Design review of the part built by this model. Coordinates are the model's own, in mm. A direction names the side the tool comes from. Give positions to 0.01 mm unless a question says otherwise; leave off trailing zeros. Loops run counter-clockwise (first coordinate to the right, second up) from the corner with the lowest first, then second, coordinate; pieces in that order, holes last. Notation, with made-up numbers: (50, -17) - (108, -17) arc R23 ccw to (108, 5) - close; hole circle Ø6 at (4.25, 31.25). An arc over 180 degrees is marked (long way). Write each question's results on one line, items separated by ' | '.
Autodesk Inventor part; units mm, degrees
ref_plane "Work Plane1" through (-19.05, 0, 0) normal (1, 0, 0) x (0, 0, -1)
ref_plane "YZ Plane" through (0, 0, 0) normal (1, 0, 0) x (0, 1, 0)
ref_plane "XZ Plane" through (0, 0, 0) normal (0, 1, 0) x (-1, 0, 0)
sketch "Sketch2" plane through (0, 0, 0) normal (1, 0, 0) x (0, 1, 0)
  circle A0 centre (0, 0) radius 3.175
  dimension "d0" = 6.35
extrude "Extrusion1" add sketch "Sketch2" along normal mid plane 127
sketch "Sketch3" plane through (-63.5, 0, 0) normal (-1, 0, 0) x (0, 0, 1)
  circle A0 centre (0, 0) radius 12.7
  dimension "d3" = 25.4
extrude "Extrusion2" add sketch "Sketch3" against normal blind 6.35
sketch "Sketch4" plane through (-57.15, 0, 0) normal (1, 0, 0) x (0, 0, -1)
  line L0 (0, 4.572) -> (1.27, 4.572)
  line L1 (1.27, 4.572) -> (1.27, 2.9099)
  circle A0 centre (0, 0) radius 3.175
  line L2 (0, -17.78) -> (0, 17.78)
  line L3 (0, 4.572) -> (-1.27, 4.572)
  line L4 (-1.27, 4.572) -> (-1.27, 2.9099)
  line L5 (-4.572, 0) -> (-4.572, -1.27)
  line L6 (-4.572, 0) -> (-4.572, 1.27)
  line L7 (-4.572, 1.27) -> (-2.9099, 1.27)
  line L8 (-4.572, -1.27) -> (-2.9099, -1.27)
  line L9 (0, -4.572) -> (1.27, -4.572)
  line L10 (0, -4.572) -> (-1.27, -4.572)
  line L11 (-1.27, -4.572) -> (-1.27, -2.9099)
  line L12 (1.27, -4.572) -> (1.27, -2.9099)
  line L13 (4.572, 0) -> (4.572, 1.27)
  line L14 (4.572, 0) -> (4.572, -1.27)
  line L15 (4.572, -1.27) -> (2.9099, -1.27)
  line L16 (4.572, 1.27) -> (2.9099, 1.27)
  arc A1 (1.27, 2.9099) -> (-1.27, 2.9099) centre (0, 0) ccw
  arc A2 (2.9099, -1.27) -> (2.9099, 1.27) centre (0, 0) ccw
  arc A3 (-2.9099, 1.27) -> (-2.9099, -1.27) centre (0, 0) ccw
  arc A4 (-1.27, -2.9099) -> (1.27, -2.9099) centre (0, 0) ccw
  dimension "d7" = 1.27
  dimension "d10" = 360
  dimension "d15" = 1.397
extrude "Extrusion3" add sketch "Sketch4" along normal blind 76.2 contours L0 L1 A0 L2 | L2 A0 L4 L3 | L2 L10 L11 A0 | A0 L12 L9 L2 | L16 L13 L14 L15 A0 | A0 L8 L5 L6 L7
ref_plane "Work Plane1" through (-19.05, 0, 0) normal (1, 0, 0) x (0, 0, -1)
sketch "Sketch5" plane through (-19.05, 0, 0) normal (1, 0, 0) x (0, 0, -1)
  circle A0 centre (0, 0) radius 3.175
  circle A1 centre (0, 0) radius 5.4209
extrude "Extrusion4" cut sketch "Sketch5" against normal blind 38.1
properties part number "ShaftForWormGear" material "PBT Plastic"
Item 1: We need section B-B on x = -26. Give the boundary of the cut face in (y, z) (3 decimals).
Output values:
outline: circle Ø6.35 at (0, 0)
Item 2: We need section C-C on z = 6.25. Give the boundary of the cut face in (x, y), then the cut area to 3 significant figures.
Output values:
outline: (-63.5, -11.06) - (-57.15, -11.06) - (-57.15, 11.06) - (-63.5, 11.06) - close | area: 140 mm²
Item 3: Tool access review of faces 1 (the face through (0, 0, -4.572)), 2 (the face through (0, 4.572, 0)), 3 (the face through (0, 0, 4.572)), 4 (the face through (4.02, 2.513, 1.94)): name each direction out of +Z, -Z, +X, -X, +Y, -Y from which nothing blocks a thin tool from reaching the whole face with its end or side.
Output values:
face 1: -Z, +X, +Y, -Y | face 2: +Z, -Z, +X, +Y | face 3: +Z, +X, +Y, -Y | face 4: none
Item 4: Wall thickness on probe 1 along X at (y, z) = (0.75, -5.5); probe 2 along X at (y, z) = (-1, 3.25); probe 3 along Z at (x, y) = (4.5, -0.75): over which ranges is each line inside the solid? List them lowest first.
Output values:
probe 1: x = -63.5 to -57.15 | probe 2: x = -63.5 to -57.15, -19.05 to 19.05 | probe 3: z = -4.57 to 4.57
Item 5: We need section A-A on y = 0. Give the boundary of the cut face in (x, z) (3 decimals).
Output values:
outline: (-63.5, -12.7) - (-57.15, -12.7) - (-57.15, -3.175) - (-19.05, -3.175) - (-19.05, -4.572) - (19.05, -4.572) - (19.05, -3.175) - (63.5, -3.175) - (63.5, 3.175) - (19.05, 3.175) - (19.05, 4.572) - (-19.05, 4.572) - (-19.05, 3.175) - (-57.15, 3.175) - (-57.15, 12.7) - (-63.5, 12.7) - close
Item 6: We need section D-D on x = 8. Give the boundary of the cut face in (y, z) (3 decimals).
Output values:
outline: (-4.572, -1.27) - (-2.91, -1.27) arc R3.175 ccw to (-1.27, -2.91) - (-1.27, -4.572) - (1.27, -4.572) - (1.27, -2.91) arc R3.175 ccw to (2.91, -1.27) - (4.572, -1.27) - (4.572, 1.27) - (2.91, 1.27) arc R3.175 ccw to (1.27, 2.91) - (1.27, 4.572) - (-1.27, 4.572) - (-1.27, 2.91) arc R3.175 ccw to (-2.91, 1.27) - (-4.572, 1.27) - close
Item 7: Clearance check with flat-ended pins moving along their axes: P1, Ø0.8, axis at x = 1, z = -3.5, coming from the -Y side; P2, Ø1.8, axis at x = -7, y = -4, coming from the -Z side; P3, Ø3, axis at x = 39.5, z = 2, coming from the -Y side. State where each tip first meets the part, or that it passes through.
Output values:
P1: stops at y = -1.27 | P2: stops at z = -1.27 | P3: stops at y = -3.14
